Answer from the drawing. Dimensions are ordinates in mm from the lowest x, y and z of the part. A direction names the side the tool comes from. Round coordinates to 2 decimals unless told otherwise and drop trailing zeros. Order: outer loops, then holes, each group sorted by start corner. A loop starts at its lowest first (then second) coordinate and runs counter-clockwise, first axis right, second up. Notation, with made-up numbers: (-6, 44) -> (12, 44) arc R14 cw to (12, 66) -> close; hole circle Ø2 at (47.25, -29). An arc over 180 degrees is marked (long way). Use a Markdown table: item, result. Add a question column.
1. Section D-D, the plane x = 71.5 is taken. Give the vertices of the cut face in (y, z) (1 decimal).
2. Section B-B, the plane x = 53 is taken. Give the vertices of the cut face in (y, z) (1 decimal).
3. Given pin 1 (10 mm diameter, centred on y = 46, z = 77, fed in from -X); pin 2 (15.5 mm diameter, centred on x = 16.5, z = 84, fed in from +Y); pin 3 (11 mm diameter, centred on x = 71, z = 84.5, fed in from -Y); pin 4 (2 mm diameter, centred on x = 62, y = 54.5, fed in from -Z), each flat-ended and moving along its own axis, determine where each tip first touches the part or whether it passes through.
4. Consider L1, parallel to Y at x = 66, z = 71.5; L2, parallel to Z at x = 48.5, y = 73; L3, parallel to Z at x = 33.5, y = 62.5. Determine where each line is inside the solid, lowest interval first. Write a range as [from, to].
5. The mould has two halves that part along X. Classify the marked faces 5, 6 and 7: +X half, -X half, draft (parallel to the pull), parting line (faces both ways), or undercut.
6. Section A-A, the plane z = 84 is taken. Give the vertices of the cut face in (x, y).
7. Section C-C, the plane y = 50 is taken. Give the vertices of the cut face in (x, z) (1 decimal).
8. For the marked faces 1, 2, 3 and 4, determine the directions among +Z, -Z, +X, -X, +Y, -Y from which every point of the face is accessible in a straight line to the end or side of a thin tool.
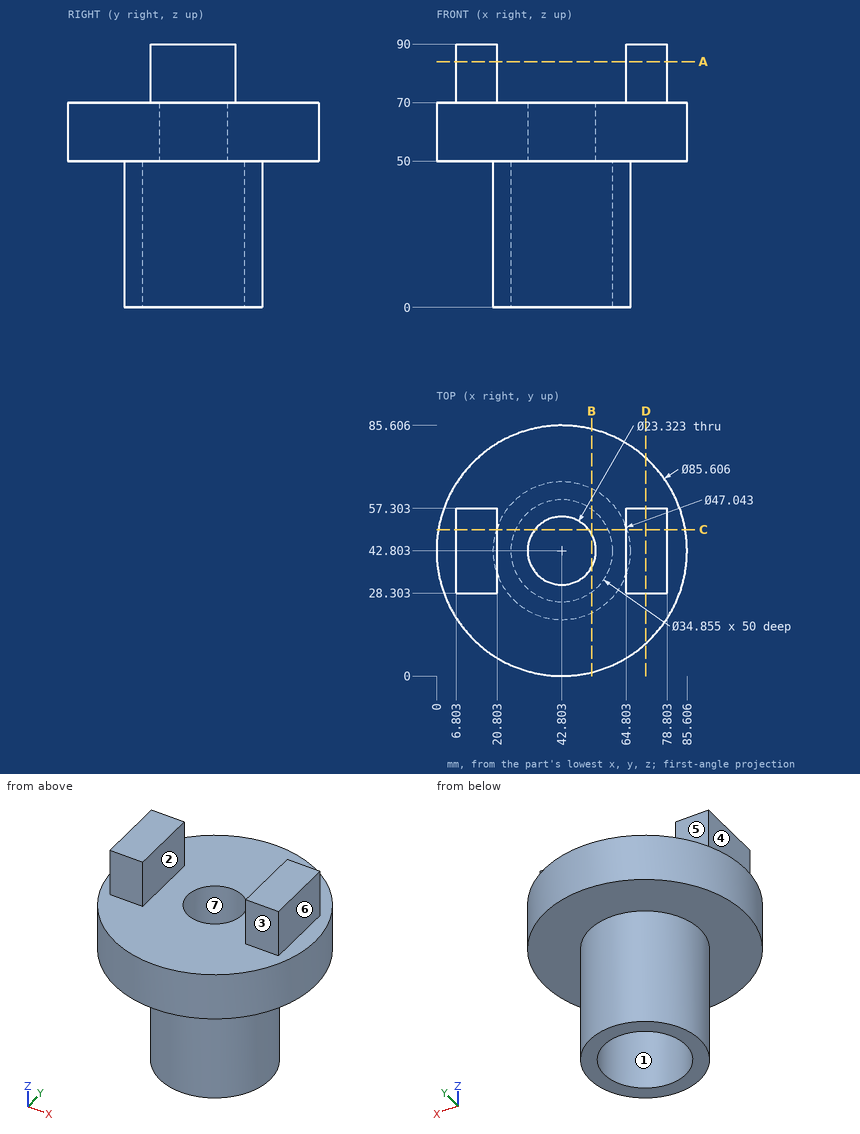
Verdict:
| question | item | result |
|---|---|---|
| 1 | outline | (11, 50) -> (74.6, 50) -> (74.6, 70) -> (57.3, 70) -> (57.3, 90) -> (28.3, 90) -> (28.3, 70) -> (11, 70) -> close |
| 2 | outline | (1.2, 50) -> (21.6, 50) -> (21.6, 0) -> (28.7, 0) -> (28.7, 50) -> (37.1, 50) -> (37.1, 70) -> (1.2, 70) -> close; (48.5, 50) -> (56.9, 50) -> (56.9, 0) -> (64, 0) -> (64, 50) -> (84.4, 50) -> (84.4, 70) -> (48.5, 70) -> close |
| 3 | pin 1 | stops at x = 6.8 |
| 3 | pin 2 | stops at y = 57.3 |
| 3 | pin 3 | stops at y = 28.3 |
| 3 | pin 4 | stops at z = 0 |
| 4 | L1 | y = [28.3, 57.3] |
| 4 | L2 | z = [50, 70] |
| 4 | L3 | z = [0, 70] |
| 5 | face 5 | draft |
| 5 | face 6 | +X half |
| 5 | face 7 | undercut |
| 6 | outline | (6.8, 28.3) -> (20.8, 28.3) -> (20.8, 57.3) -> (6.8, 57.3) -> close; (64.8, 28.3) -> (78.8, 28.3) -> (78.8, 57.3) -> (64.8, 57.3) -> close |
| 7 | outline | (0.6, 50) -> (20.4, 50) -> (20.4, 0) -> (26.9, 0) -> (26.9, 50) -> (33.6, 50) -> (33.6, 70) -> (20.8, 70) -> (20.8, 90) -> (6.8, 90) -> (6.8, 70) -> (0.6, 70) -> close; (52, 50) -> (58.7, 50) -> (58.7, 0) -> (65.2, 0) -> (65.2, 50) -> (85, 50) -> (85, 70) -> (78.8, 70) -> (78.8, 90) -> (64.8, 90) -> (64.8, 70) -> (52, 70) -> close |
| 8 | face 1 | -Z |
| 8 | face 2 | +Z, +Y, -Y |
| 8 | face 3 | +Z, +X, -X, -Y |
| 8 | face 4 | +Z, -X, +Y, -Y |
